Input: part model. Units: mm. Frame: model coordinates. A direction names the side the tool comes from. Give positions to 0.01 mm unless a question says otherwise; leave off trailing zeros. Use CSV: the item, a comma, the result in double quotes. Start each with the question number.
Q1. Material intervals for line 1 along Y through (x, z) = (-16.5, 16.75); line 2 along Y through (x, z) = (5.5, 14.5); line 3 along X through (y, z) = (-1, 18.75), sorted ascending.
Q2. Pin query (flat end, axial travel): pin 1 (1.2 mm diameter, centred on x = 16, y = 21.5, fed in from +Z); pin 2 (2.5 mm diameter, centred on x = 16.5, y = 10.5, fed in from +Z); pin 3 (6.5 mm diameter, centred on x = -5.5, y = 0, fed in from +Z); pin 4 (4.5 mm diameter, centred on x = 17.5, y = -21, fed in from +Z). Return the tip coordinate at first contact, or that it passes through.
Q3. Reachability of faces 1 (the flat face through (21, 11, 0)), 2 (the flat face through (-17, 11, 10)) from +Z, -Z, +X, -X, +Y, -Y: full face, straight path, thin tool, end or side. Return the list, or none.
Q4. Section A-A, the plane z = 21.5. State how many separate pieces and enclosed holes the cut face has, plus the area to 3 significant figures.
Q5. Pull-direction query (X, two-part tool) for faces 3 (the cylindrical face through (-2.88, -10.17, 17.1)), 4 (the flat face through (-24, 49, 11)), 5 (the flat face through (21, -29, 24)); classes: released by +X, released by -X, zero draft, split by the parting line, or undercut.
from build123d import *

# Parameters (mm, degrees)
SKETCH_W        = 93
SKETCH_H        = 80
PAD_DEPTH       = 25
SKETCH001_R     = 3.5
SKETCH001_R_2   = 3
SKETCH001_R_3   = 2.75
SKETCH001_R_4   = 2.5
SKETCH001_R_5   = 2.4
SKETCH001_R_6   = 2
SKETCH001_R_7   = 1.5
POCKET_DEPTH    = 15
CHAMFER_SIZE    = 2
CHAMFER001_SIZE = 1


with BuildPart() as part:
    # Sketch → Pad (new body)
    with BuildSketch(Plane.XY):
        with Locations((21.5, 10)):
            Rectangle(SKETCH_W, SKETCH_H)
    extrude(amount=PAD_DEPTH)

    # Sketch001 (on Face6 of Pad) → Pocket (cut)
    with BuildSketch(Plane.XY.offset(25)):
        with Locations((-16.5, -22)):
            Circle(SKETCH001_R)
        with Locations((-16.5, -11)):
            Circle(SKETCH001_R)
        with Locations((-16.5, 0)):
            Circle(SKETCH001_R)
        with Locations((-16.5, 11)):
            Circle(SKETCH001_R_2)
        with Locations((-5.5, -22)):
            Circle(SKETCH001_R_3)
        with Locations((-5.5, -11)):
            Circle(SKETCH001_R_3)
        with Locations((-5.5, 0)):
            Circle(SKETCH001_R_3)
        with Locations((-5.5, 11)):
            Circle(SKETCH001_R_4)
        with Locations((5.5, -22)):
            Circle(SKETCH001_R_5)
        with Locations((5.5, -11)):
            Circle(SKETCH001_R_5)
        with Locations((5.5, 0)):
            Circle(SKETCH001_R_5)
        with Locations((5.5, 11)):
            Circle(SKETCH001_R_6)
        with Locations((16.5, -22)):
            Circle(SKETCH001_R_6)
        with Locations((16.5, -11)):
            Circle(SKETCH001_R_6)
        with Locations((16.5, 0)):
            Circle(SKETCH001_R_6)
        with Locations((16.5, 11)):
            Circle(SKETCH001_R_7)
        with Locations((-16.5, 22)):
            Circle(SKETCH001_R)
        with Locations((-5.5, 22)):
            Circle(SKETCH001_R_2)
        with Locations((5.5, 22)):
            Circle(SKETCH001_R_4)
        with Locations((16.5, 22)):
            Circle(SKETCH001_R_6)
    extrude(amount=-POCKET_DEPTH, mode=Mode.SUBTRACT)

    # Chamfer
    chamfer_edges = [part.edges().sort_by_distance(p)[0] for p in [
        (68, -30, 12.5),
        (-25, -30, 12.5),
        (-25, 10, 25),
        (21.5, -30, 25),
        (68, 10, 25),
        (68, 50, 12.5),
        (21.5, 50, 25),
        (-25, 50, 12.5),
    ]]
    chamfer(chamfer_edges, length=CHAMFER_SIZE)

    # Chamfer001
    chamfer001_edges = [part.edges().sort_by_distance(p)[0] for p in [
        (-20, -22, 25),
        (-8.25, -22, 25),
        (3.1, -22, 25),
        (14.5, -22, 25),
        (14.5, -11, 25),
        (14.5, 0, 25),
        (15, 11, 25),
        (14.5, 22, 25),
        (3, 22, 25),
        (3.5, 11, 25),
        (3.1, 0, 25),
        (3.1, -11, 25),
        (-8.25, -11, 25),
        (-8.25, 0, 25),
        (-8, 11, 25),
        (-8.5, 22, 25),
        (-20, 22, 25),
        (-19.5, 11, 25),
        (-20, 0, 25),
        (-20, -11, 25),
    ]]
    chamfer(chamfer001_edges, length=CHAMFER001_SIZE)


solid = part.part
A:
1,line 1,"-30 to -25.5, -18.5 to -14.5, -7.5 to -3.5, 3.5 to 8, 14 to 18.5, 25.5 to 50"
1,line 2,"-30 to -24.4, -19.6 to -13.4, -8.6 to -2.4, 2.4 to 9, 13 to 19.5, 24.5 to 50"
1,line 3,"-25 to -19.85, -13.15 to -8.06, -2.94 to 3.32, 7.68 to 14.77, 18.23 to 68"
2,pin 1,"z = 10"
2,pin 2,"z = 24.25"
2,pin 3,"z = 24.5"
2,pin 4,"z = 25"
3,face 1,"-Z, +X, -X, +Y, -Y"
3,face 2,"+Z"
4,separate pieces,"1"
4,enclosed holes,"20"
4,area,"6,990 mm^2"
5,face 3,"undercut"
5,face 4,"released by -X"
5,face 5,"zero draft"
